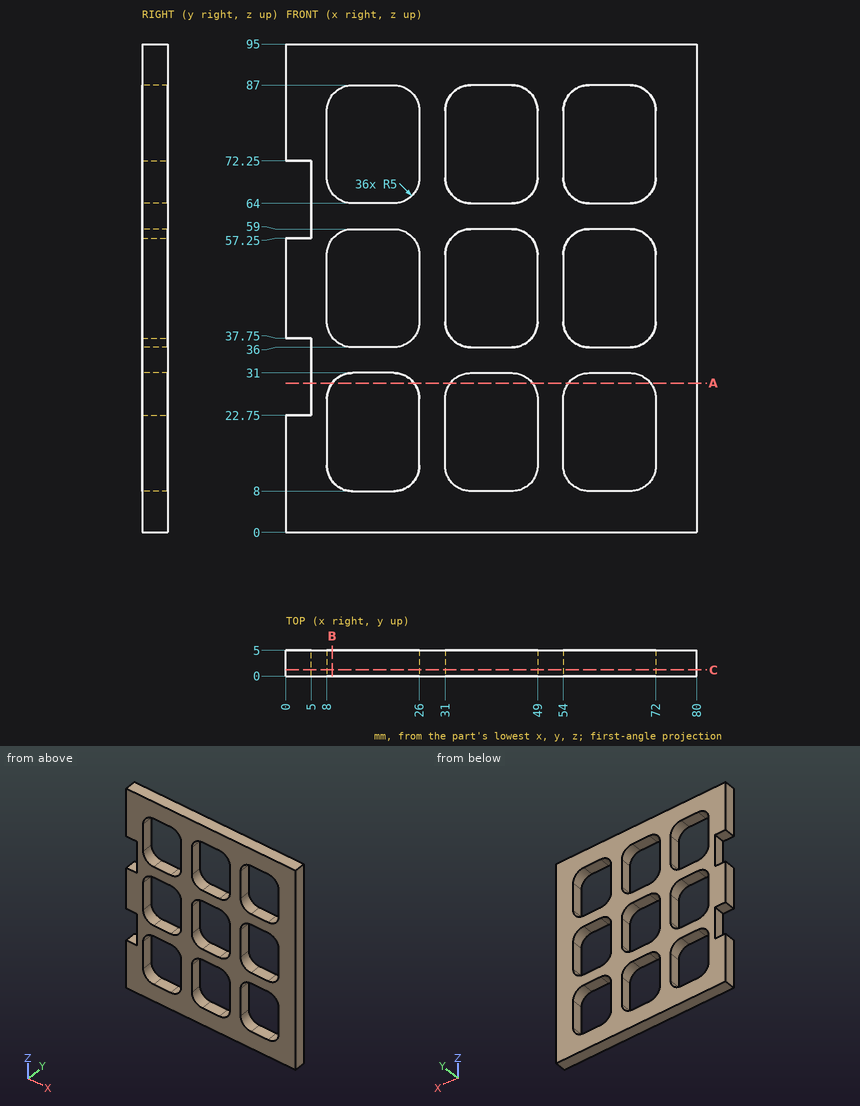
Geometry check sheet. Reference: drawing and pictorial views, mm from the part's lowest x, y, z. Round coordinates to 2 decimals unless told otherwise and drop trailing zeros. Write each loop counter-clockwise with the first axis right and the second up, starting at its lowest first coordinate (ties: lowest second). Pieces come first, ordered by that corner, then holes. Notation, with made-up numbers: (-39.75, 42) -> (-11.75, 42) arc R30 ccw to (-11.75, 69) -> close; hole circle Ø4 at (21, -21). An arc over 180 degrees is marked (long way). One line per question, with ' | ' between items. Start each with the question number.
1. Scan lines: line 1 along Z through (x, y) = (37, 0.8); line 2 along X through (y, z) = (1.8, 43.5); line 3 along X through (y, z) = (0.8, 39.5). Record each from-to range of solid material in increasing order. Write a range as from..to.
2. Sectioned sample at C-C, the plane y = 1.2. Count the separate pieces of the cut face and the enclosed holes in it, then the cut area to 3 significant figures.
3. Sectioned sample at A-A, the plane z = 29. Record the cut outline in (x, y), then the cut area to 3 significant figures.
4. Sectioned sample at B-B, the plane x = 9. Record the cut outline in (y, z), then the cut area to 3 significant figures.
Taken from the geometry:
1) line 1: z = 0..8, 31..36, 59..64, 87..95 | line 2: x = 0..8, 26..31, 49..54, 72..80 | line 3: x = 0..8.23, 25.77..31.23, 48.77..54.23, 71.77..80
2) separate pieces: 1 | enclosed holes: 9 | area: 3,920 mm^2
3) outline: (5, 0) -> (9, 0) -> (9, 5) -> (5, 5) -> close; (25, 0) -> (32, 0) -> (32, 5) -> (25, 5) -> close; (48, 0) -> (55, 0) -> (55, 5) -> (48, 5) -> close; (71, 0) -> (80, 0) -> (80, 5) -> (71, 5) -> close | area: 135 mm^2
4) outline: (0, 0) -> (5, 0) -> (5, 10) -> (0, 10) -> close; (0, 29) -> (5, 29) -> (5, 38) -> (0, 38) -> close; (0, 57) -> (5, 57) -> (5, 66) -> (0, 66) -> close; (0, 85) -> (5, 85) -> (5, 95) -> (0, 95) -> close | area: 190 mm^2
